Geometry check sheet. Reference: the model listing, model coordinates, mm. Face numbers are marked on the shaded views. A direction names the side the tool comes from. Coordinates: 2 decimals unless noted, no trailing zeros. Write each loop counter-clockwise with the first axis right and the second up, starting at its lowest first coordinate (ties: lowest second). Pieces come first, ordered by that corner, then holes. Notation, with made-up numbers: (-38.75, 35) -> (-28.75, 35) arc R16 cw to (-28.75, 46) -> close; hole circle Ø1 at (-24.75, -17). An arc over 180 degrees is marked (long way). Answer in a Markdown table with one row per item. Add a question column.
1. Cross-section at D-D on x = 41. Record the cut outline in (y, z) (3 decimals), and give its area (3 significant figures).
2. Cross-section at B-B on z = 31.5. Record the cut outline in (x, y) (3 decimals).
3. Set-up check for the marked faces 1, 2 and 3: record each of +Z, -Z, +X, -X, +Y, -Y from which the full face is reachable in a straight line by a thin tool's end or side.
4. Scan lines: L1, parallel to Y at x = 30, z = 79; L2, parallel to X at y = 15, z = 53 (3 decimals); L3, parallel to X at y = 6.25, z = 0.5. Record each from-to range of solid material in increasing order. Write a range as from..to.
5. Cross-section at A-A on x = -52. Record the cut outline in (y, z) (3 decimals), and give its area (3 significant figures).
6. Depth check by flat-ended pin: P1, Ø3, axis at y = 4, z = 20.5, coming from the -X side; P2, Ø6, axis at y = 13.5, z = 52, coming from the -X side; P3, Ø1.9, axis at x = -1.5, z = -84.5, coming from the +Y side; P4, Ø6, axis at x = -42.5, z = 31.5, coming from the -Y side. Enter the tip coordinate at first touch or a pass-through.
7. Cross-section at C-C on y = 4.5. Record the cut outline in (x, z) (3 decimals).
```python
from build123d import *

# Parameters (mm, degrees)
SKETCH1_R           = 85.725
BOSS_EXTRUDE1_DEPTH = 12.7
BOSS_EXTRUDE2_DEPTH = 6.35
SKETCH3_R           = 6.35
SKETCH3_R_2         = 5.08
BOSS_EXTRUDE3_DEPTH = 6.096


with BuildPart() as part:
    # Sketch1 → Boss-Extrude1 (new body)
    with BuildSketch(Plane(origin=(0, 0, 0), x_dir=(1, 0, 0), z_dir=(0, 1, 0))):
        Circle(SKETCH1_R)
    extrude(amount=BOSS_EXTRUDE1_DEPTH)

    # Sketch2 → Boss-Extrude2 (add)
    with BuildSketch(Plane(origin=(0, 12.7, 0), x_dir=(1, 0, 0), z_dir=(0, 1, 0))):
        Polygon((-25.4, 81.875610685), (25.4, 81.875610685), (85.725, 0), (0, -85.725), (-85.725, 0), align=None)
    extrude(amount=BOSS_EXTRUDE2_DEPTH)

    # Sketch3 → Boss-Extrude3 (add)
    with BuildSketch(Plane(origin=(0, 12.7, 0), x_dir=(1, 0, 0), z_dir=(0, 1, 0))):
        with Locations((-51.739614409, -51.739614409)):
            Circle(SKETCH3_R)
        with Locations((51.739614409, -51.739614409)):
            Circle(SKETCH3_R)
        with Locations((62.288840877, 45.893695259)):
            Circle(SKETCH3_R_2)
        with Locations((-62.288840877, 45.893695259)):
            Circle(SKETCH3_R_2)
    extrude(amount=BOSS_EXTRUDE3_DEPTH)


solid = part.part
```
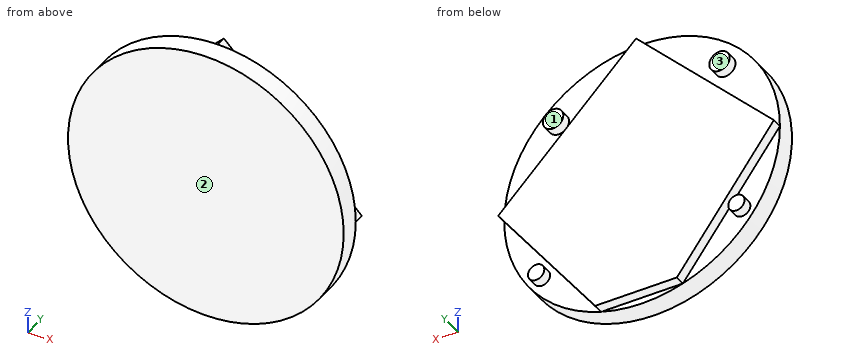
Results found:
| question | item | result |
|---|---|---|
| 1 | outline | (0, -75.285) -> (12.7, -75.285) -> (12.7, -60.703) -> (19.05, -60.703) -> (19.05, 44.725) -> (12.7, 44.725) -> (12.7, 75.285) -> (0, 75.285) -> close |
| 1 | area | 2,580 mm^2 |
| 2 | outline | (-79.728, 0) -> (79.728, 0) -> (79.728, 12.7) -> (54.225, 12.7) -> (54.225, 19.05) -> (-54.225, 19.05) -> (-54.225, 12.7) -> (-79.728, 12.7) -> close |
| 3 | face 1 | +Z, +X, +Y |
| 3 | face 2 | +Z, -Z, +X, -X, -Y |
| 3 | face 3 | +Z, -X, +Y |
| 4 | L1 | y = 0..12.7 |
| 4 | L2 | x = -57.963..-45.516, -32.725..32.725, 45.516..57.963 |
| 4 | L3 | x = -85.72..85.72 |
| 5 | outline | (0, -68.153) -> (12.7, -68.153) -> (12.7, -45.773) -> (19.05, -45.773) -> (19.05, 33.725) -> (12.7, 33.725) -> (12.7, 45.395) -> (18.796, 45.395) -> (18.796, 58.084) -> (12.7, 58.084) -> (12.7, 68.153) -> (0, 68.153) -> close |
| 5 | area | 2,310 mm^2 |
| 6 | P1 | stops at x = -83.59 |
| 6 | P2 | stops at x = -70.26 |
| 6 | P3 | stops at y = 12.7 |
| 6 | P4 | stops at y = 0 |
| 7 | outline | circle Ø171.45 at (0, 0) |
